from build123d import *

# Parameters (mm, degrees)
F1_DEPTH = 93.98
F3_START = -2.159
F3_DEPTH = 2.54
F4_R     = 0.508


with BuildPart() as f1:
    # F0 (on Front) → F1 (new body)
    with BuildSketch(Plane.XZ):
        with BuildLine():
            ThreePointArc((-31.1404, 0), (0, 31.1404), (31.1404, 0))
            Line((31.1404, 0), (31.1404, -2.159))
            Line((31.1404, -2.159), (34.036, -2.159))
            Line((34.036, -2.159), (34.036, 0))
            ThreePointArc((34.036, 0), (0, 34.036), (-34.036, 0))
            Line((-34.036, 0), (-34.036, -2.159))
            Line((-34.036, -2.159), (-31.1404, -2.159))
            Line((-31.1404, -2.159), (-31.1404, 0))
        make_face()
    extrude(amount=F1_DEPTH)

    # F2 (on Top) → F3 (join)
    with BuildSketch(Plane.XY.offset(F3_START)):
        Polygon((-31.1404, -29.21), (-31.1404, -17.526), (-28.1178, -17.526), (-28.1178, -5.588), (-31.1404, -5.588), (-31.1404, 0), (-34.036, 0), (-34.036, -93.98), (-31.1404, -93.98), (-31.1404, -88.392), (-28.1178, -88.392), (-28.1178, -76.454), (-31.1404, -76.454), (-31.1404, -64.77), (-28.1178, -64.77), (-28.1178, -52.832), (-31.1404, -52.832), (-31.1404, -41.148), (-28.1178, -41.148), (-28.1178, -29.21), align=None)
        Polygon((28.1178, -17.526), (31.1404, -17.526), (31.1404, -29.21), (28.1178, -29.21), (28.1178, -41.148), (31.1404, -41.148), (31.1404, -52.832), (28.1178, -52.832), (28.1178, -64.77), (31.1404, -64.77), (31.1404, -76.454), (28.1178, -76.454), (28.1178, -88.392), (31.1404, -88.392), (31.1404, -93.98), (34.036, -93.98), (34.036, 0), (31.1404, 0), (31.1404, -5.588), (28.1178, -5.588), align=None)
    extrude(amount=-F3_DEPTH)

    # F4
    f4_edges = [f1.edges().sort_by_distance(p)[0] for p in [
        (0, -93.98, 31.1404),
        (31.1404, -93.98, -2.3495),
        (32.5882, -93.98, -4.699),
        (34.036, -93.98, -2.3495),
        (0, -93.98, 34.036),
        (-34.036, -93.98, -2.3495),
        (-32.5882, -93.98, -4.699),
        (-31.1404, -93.98, -2.3495),
        (0, 0, 31.1404),
        (31.1404, 0, -2.3495),
        (32.5882, 0, -4.699),
        (34.036, 0, -2.3495),
        (0, 0, 34.036),
        (-34.036, 0, -2.3495),
        (-32.5882, 0, -4.699),
        (-31.1404, 0, -2.3495),
        (34.036, -46.99, -4.699),
        (-34.036, -46.99, -4.699),
    ]]
    fillet(f4_edges, radius=F4_R)


solid = f1.part
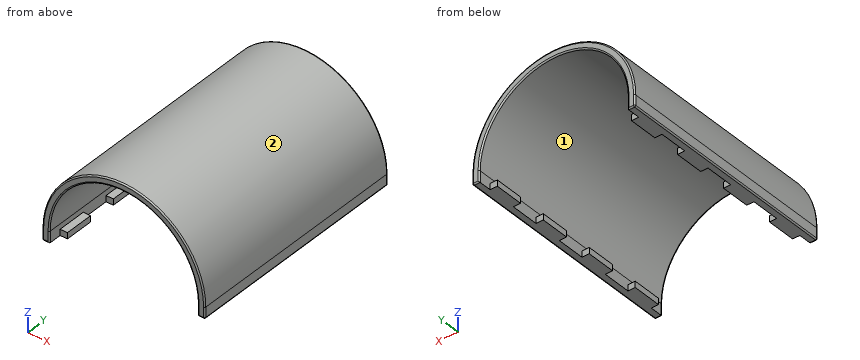
Build history of the part. All positions in model axes, mm. Face numbers are marked on the shaded views. Coordinates: 2 decimals unless noted, no trailing zeros. Write each loop counter-clockwise with the first axis right and the second up, starting at its lowest first coordinate (ties: lowest second). Pieces come first, ordered by that corner, then holes. Notation, with made-up numbers: (-4.5, 81.5) -> (32.5, 81.5) arc R10 cw to (32.5, 85.5) -> close; hole circle Ø8 at (45, 65). An arc over 180 degrees is marked (long way). Use CSV: the item, a comma, the result in double quotes. Start each with the question number.
Q1. Drill centre lines: probe 1 along X at (y, z) = (-32, -1); probe 2 along X at (y, z) = (-60.5, 5); probe 3 along Z at (x, y) = (0, -77). Where is each one in solid material? Low to high.
Q2. Cut at C-C, the plane y = -58.5. List the corners of the cut face in (x, z).
Q3. Pull direction Z, two halves, no side cores. Call the marked faces 1 and 2: released by +Z, released by -Z, zero draft, split by the parting line, or undercut.
Q4. Flat gauge pins, fed straight in: pin 1 Ø1.5 at (y, z) = (-34.5, 5.5) entering from -X; pin 2 Ø2.5 at (x, y) = (-30, -56) entering from +Z; pin 3 Ø6 at (y, z) = (-80.5, 14.5) entering from +X. Where does each tip first touch, or does it go through?
Q5. Cut at A-A, the plane z = -1. List the corners of the cut face in (x, y).
Q6. Cut at B-B, the plane x = 0. List the corners of the cut face in (y, z), then the cut area to 3 significant figures.
Checked values:
1,probe 1,"x = -34.04 to -31.14, 31.14 to 34.04"
1,probe 2,"x = -33.67 to -30.74, 30.74 to 33.67"
1,probe 3,"z = 31.14 to 34.04"
2,outline,"(-34.04, -4.19) arc R0.51 ccw to (-33.53, -4.7) -> (-28.12, -4.7) -> (-28.12, -2.16) -> (-31.14, -2.16) -> (-31.14, 0) arc R31.14 cw to (31.14, 0) -> (31.14, -2.16) -> (28.12, -2.16) -> (28.12, -4.7) -> (33.53, -4.7) arc R0.51 ccw to (34.04, -4.19) -> (34.04, 0) arc R34.04 ccw to (-34.04, 0) -> close"
3,face 1,"undercut"
3,face 2,"released by +Z"
4,pin 1,"stops at x = -33.7"
4,pin 2,"stops at z = 18.22"
4,pin 3,"stops at x = 32.03"
5,outline,"(-34.04, -93.47) arc R0.51 ccw to (-33.53, -93.98) -> (-31.65, -93.98) arc R0.51 ccw to (-31.14, -93.47) -> (-31.14, -0.51) arc R0.51 ccw to (-31.65, 0) -> (-33.53, 0) arc R0.51 ccw to (-34.04, -0.51) -> close; (31.14, -93.47) arc R0.51 ccw to (31.65, -93.98) -> (33.53, -93.98) arc R0.51 ccw to (34.04, -93.47) -> (34.04, -0.51) arc R0.51 ccw to (33.53, 0) -> (31.65, 0) arc R0.51 ccw to (31.14, -0.51) -> close"
6,outline,"(-93.98, 31.65) arc R0.51 ccw to (-93.47, 31.14) -> (-0.51, 31.14) arc R0.51 ccw to (0, 31.65) -> (0, 33.53) arc R0.51 ccw to (-0.51, 34.04) -> (-93.47, 34.04) arc R0.51 ccw to (-93.98, 33.53) -> close"
6,area,"272 mm²"
